The drawing under review shows one solid part. Ordinate dimensions are in mm from its lowest x, y, z. A direction names the side the tool comes from. Give positions to 0.01 mm unless a question says otherwise; leave off trailing zeros. Loops run counter-clockwise (first coordinate to the right, second up) from the corner with the lowest first, then second, coordinate; pieces in that order, holes last. Notation, with made-up numbers: M 70,85.25 L 102,85.25 A21 ccw 102,92.25 Z; hole C 34.5,62.25 d5. An arc over 180 degrees is marked long. Write item = value, one per line. Start each with the question number.
1. We need section D-D on x = 20.75. Give the boundary of the cut face in (y, z).
2. We need section B-B on y = 2.75. Give the boundary of the cut face in (x, z), then the cut area to 3 significant figures.
3. For pin 1 (4 mm diameter, centred on x = 9, z = 10, fed in from +Y); pin 2 (1.5 mm diameter, centred on x = 18.5, z = 4.5, fed in from -Y); pin 3 (1.3 mm diameter, centred on y = 1.5, z = 10.5, fed in from +X), all flat-tipped, find the tip position at first contact; note any pin that passes through.
4. We need section C-C on z = 8. Give the boundary of the cut face in (x, y).
5. For the marked faces 1, 2, 3 and 4, list the 3-axis set-ups (+Z, -Z, +X, -X, +Y, -Y) from which the entire face can be reached by the end or side of a thin tool; tool diameter is ignored.
6. We need section A-A on x = 11. Give the boundary of the cut face in (y, z).
7. Draft analysis for pull direction Z (two halves, no side actions). For the marked faces 5, 6 and 7, state which applies: pulls with the +Z half, pulls with the -Z half, needs draft (parallel to the pull), parting line crosses it, or undercut.
8. Wall thickness on line 1 along X through (y, z) = (7.75, 2); line 2 along Z through (x, y) = (21, 2.5); line 3 along Z through (x, y) = (11, 0.5): over which ranges is each line inside the solid? List them lowest first. Write a range as from..to.
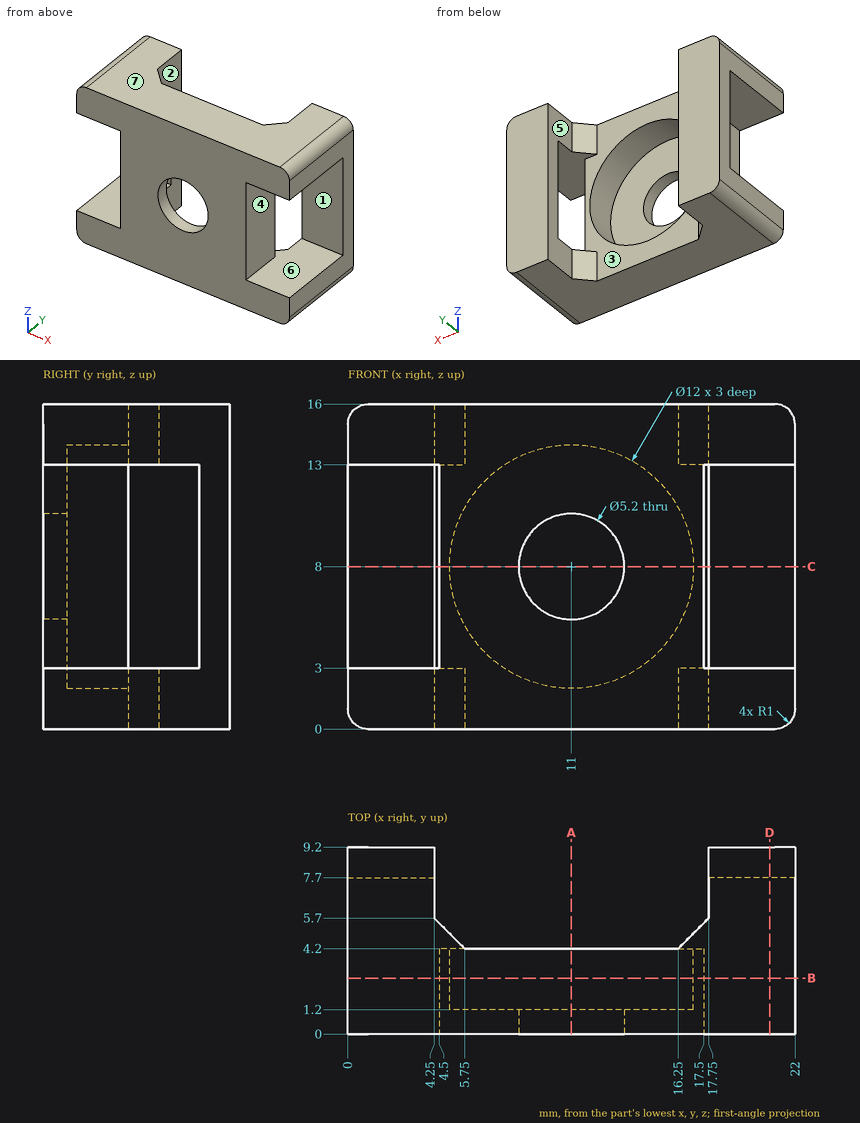
Final values:
q1.outline = M 0,0 L 9.2,0 L 9.2,16 L 0,16 L 0,13 L 7.7,13 L 7.7,3 L 0,3 Z
q2.outline = M 0,1 A1 ccw 1,0 L 21,0 A1 ccw 22,1 L 22,3 L 17.5,3 L 17.5,13 L 22,13 L 22,15 A1 ccw 21,16 L 1,16 A1 ccw 0,15 L 0,13 L 4.5,13 L 4.5,3 L 0,3 Z; hole C 11,8 d12
q2.area = 148 mm²
q3.pin_1 = 1.2
q3.pin_2 = 7.7
q3.pin_3 = 17.5
q4.outline = M 0,7.7 L 4.25,7.7 L 4.25,9.2 L 0,9.2 Z; M 4.5,0 L 8.4,0 L 8.4,1.2 L 5,1.2 L 5,4.2 L 4.5,4.2 Z; M 13.6,0 L 17.5,0 L 17.5,4.2 L 17,4.2 L 17,1.2 L 13.6,1.2 Z; M 17.75,7.7 L 22,7.7 L 22,9.2 L 17.75,9.2 Z
q5.face_1 = +X, -X, -Y
q5.face_2 = +Z, -Z, +Y
q5.face_3 = +Y
q5.face_4 = +X, +Y, -Y
q6.outline = M 0,0 L 4.2,0 L 4.2,2 L 1.2,2 L 1.2,5.4 L 0,5.4 Z; M 0,10.6 L 1.2,10.6 L 1.2,14 L 4.2,14 L 4.2,16 L 0,16 Z
q7.face_5 = needs draft
q7.face_6 = undercut
q7.face_7 = pulls with the +Z half
q8.line_1 = 0..4.25, 17.75..22
q8.line_2 = 0..3, 13..16
q8.line_3 = 0..5.4, 10.6..16
